Part model, mm, in its own coordinate system. Face numbers are marked on the shaded views. Give positions to 0.01 mm unless a question says otherwise; leave off trailing zeros. Order: outer loops, then holes, each group sorted by start corner. A loop starts at its lowest first (then second) coordinate and runs counter-clockwise, first axis right, second up. Notation, with made-up numbers: (72.25, -33.75) -> (121.25, -33.75) arc R29 cw to (121.25, -9.75) -> close; hole circle Ø7 at (5.5, 58.5). An arc over 180 degrees is marked (long way). Write item = value, one per line. Start each with the question number.
Item 1: Drill centre lines: line 1 along X through (y, z) = (6.5, 25); line 2 along X through (y, z) = (-4, 29); line 3 along Y through (x, z) = (15, 38.5). Where is each one in solid material? Low to high.
Item 2: Flat gauge pins, fed straight in: P1, Ø5, axis at y = -8, z = 22.5, coming from the +X side; P2, Ø8, axis at x = 0.5, z = 22.5, coming from the +Y side; P3, Ø4, axis at x = -13, z = 31, coming from the -Y side. Where does each tip first touch, or does it go through?
Item 3: Band-saw the part on A-A on y = 0. Write the cut outline in (x, z), plus the area to 3 significant figures.
Item 4: Band-saw the part on C-C on z = 6. Write the cut outline in (x, y), plus the area to 3 significant figures.
Item 5: Band-saw the part on D-D on z = 11. Write the cut outline in (x, y).
Item 6: Pull direction Y, two halves, no side cores. Call the marked faces 1, 2 and 3: +Y half, -Y half, draft (parallel to the pull), parting line (faces both ways), or undercut.
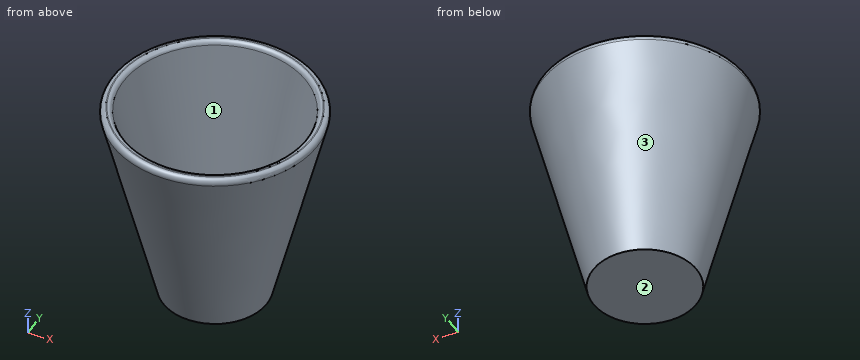
```python
from build123d import *

# Parameters (mm, degrees)
FILLET_R = 1


with BuildPart() as cono001:
    # Cone001 → Cone001 (revolve)
    with BuildSketch(Plane(origin=(0, 0, 1), x_dir=(1, 0, 0), z_dir=(0, -1, 0))):
        Polygon((0, 0), (8, 0), (18, 40), (0, 40), align=None)
    revolve(axis=Axis((0, 0, 1), (0, 0, 1)))


with BuildPart() as fillet_body:
    # Cone → Cone (revolve)
    with BuildSketch(Plane.XZ):
        Polygon((0, 0), (10, 0), (20, 40), (0, 40), align=None)
    revolve(axis=Axis((0, 0, 0), (0, 0, 1)))

    # Cut: cut Cono001
    add(cono001.part, mode=Mode.SUBTRACT)

    # Fillet
    fillet_edges = [fillet_body.edges().sort_by_distance(p)[0] for p in [
        (-20, 0, 40),
        (-17.75, 0, 40),
    ]]
    fillet(fillet_edges, radius=FILLET_R)


solid = fillet_body.part
```
Values found:
q1.line_1 = -14.89 to -12.4, 12.4 to 14.89
q1.line_2 = -16.78 to -14.46, 14.46 to 16.78
q1.line_3 = -12.65 to -8.77, 8.77 to 12.65
q2.P1 = 14.83
q2.P2 = 16.62
q2.P3 = -14.05
q3.outline = (-19.69, 38.76) -> (-10, 0) -> (10, 0) -> (19.69, 38.76) arc R1 ccw to (18.72, 40) -> (18.53, 40) arc R1 ccw to (17.56, 39.24) -> (8, 1) -> (-8, 1) -> (-17.56, 39.24) arc R1 ccw to (-18.53, 40) -> (-18.72, 40) arc R1 ccw to start
q3.area = 195 mm^2
q4.outline = circle Ø23 at (0, 0); hole circle Ø18.5 at (0, 0)
q4.area = 147 mm^2
q5.outline = circle Ø25.5 at (0, 0); hole circle Ø21 at (0, 0)
q6.face_1 = undercut
q6.face_2 = draft
q6.face_3 = parting line
